Autodesk Inventor part; units mm, degrees
ref_plane "YZ Plane" through (0, 0, 0) normal (1, 0, 0) x (0, 1, 0)
ref_plane "XZ Plane" through (0, 0, 0) normal (0, 1, 0) x (-1, 0, 0)
ref_plane "XY Plane" through (0, 0, 0) normal (0, 0, 1) x (1, 0, 0)
sketch "Sketch1" plane through (0, 0, 0) normal (0, 0, 1) x (1, 0, 0)
  circle A0 centre (0, 0) radius 4.445
  dimension "d0" = 8.89
extrude "Extrusion1" add sketch "Sketch1" along normal blind 1.27
sketch "Sketch2" plane through (0, 0, 0) normal (0, 0, -1) x (-1, 0, 0)
  circle A0 centre (0, 0) radius 4.445
  circle A1 centre (0, 0) radius 1.27
  dimension "d3" = 2.54
extrude "Extrusion2" add sketch "Sketch2" along normal blind 1.27 contours A1
sketch "Sketch3" plane through (0, 0, 1.27) normal (0, 0, 1) x (1, 0, 0)
  circle A0 centre (0, 0) radius 4.445
  circle A1 centre (0, 0) radius 3.175
  dimension "d6" = 6.35
extrude "Extrusion3" add sketch "Sketch3" along normal blind 1.27 contours A1
sketch "Sketch4" plane through (0, 0, 2.54) normal (0, 0, 1) x (1, 0, 0)
  circle A0 centre (0, 0) radius 3.175
  line L0 (6.35, -9.525) -> (6.35, 9.525)
  line L1 (4.9582, 9.1002) -> (-14.9068, 3.0367)
  line L2 (-14.9068, -3.0367) -> (4.9582, -9.1002)
  arc A1 (7.808, -8.5899) -> (7.808, 8.5899) centre (1.27, 0) ccw
  arc A2 (-14.9068, 3.0367) -> (-14.9068, -3.0367) centre (-13.9799, 0) ccw
  arc A3 (7.808, 8.5899) -> (4.9582, 9.1002) centre (5.8851, 6.0635) ccw
  arc A4 (4.9582, -9.1002) -> (7.808, -8.5899) centre (5.8851, -6.0635) ccw
  point P0 (-24.8555, 0)
  dimension "d9" = 19.05
  dimension "d13" = 9.525
  dimension "d14" = 6.35
  dimension "d15" = 10.795
  dimension "d16" = 3.175
  dimension "d20" = 0
  dimension "d21" = 22.225
  dimension "d22" = 3.175
extrude "Extrusion4" add sketch "Sketch4" along normal blind 3.81 contours A0 | A4 L2 A2 L1 A3 L0 | L0 A3 A1 A4
properties part number "Knob 1764"
Check sheet for the modelled part. Datum: model origin and axes. Units: mm. A direction names the side the tool comes from. Round coordinates to 2 decimals unless told otherwise and drop trailing zeros. Write each loop counter-clockwise with the first axis right and the second up, starting at its lowest first coordinate (ties: lowest second). Pieces come first, ordered by that corner, then holes. Notation, with made-up numbers: (18, -8) - (29, -8) arc R31 ccw to (29, 24) - close; hole circle Ø10 at (58.5, 32.5). An arc over 180 degrees is marked (long way). Return JSON: item names as keys, results as strings.
Q1. Cross-section at B-B (y = 0). Record the boundary of the cut face in (x, z) (3 decimals).
Returned:
{"outline": "(-17.155, 2.54) - (-3.175, 2.54) - (-3.175, 1.27) - (-4.445, 1.27) - (-4.445, 0) - (-1.27, 0) - (-1.27, -1.27) - (1.27, -1.27) - (1.27, 0) - (4.445, 0) - (4.445, 1.27) - (3.175, 1.27) - (3.175, 2.54) - (12.065, 2.54) - (12.065, 6.35) - (-17.155, 6.35) - close"}
Q2. Depth check by flat-ended pin: P1, Ø1.5, axis at x = -5.5, y = -4, coming from the -Z side; P2, Ø4, axis at x = -5.5, y = 6.5, coming from the +Z side; P3, Ø8, axis at x = 0, y = 7, coming from the -Z side; P4, Ø1, axis at x = -12.5, z = 0.5, coming from the +Y side. Enter the tip coordinate at first touch or a pass-through.
Returned:
{"P1": "stops at z = 2.54", "P2": "stops at z = 6.35", "P3": "stops at z = 0", "P4": "passes through"}
Q3. Access from +Z, -Z, +X, -X, +Y, -Y to the whole of each face (thin tool, end or side, straight path). Record for faces 1 (the flat face through (-1.1, -0.9, 0)), 2 (the cylindrical face through (12.064, 0.139, 4.418)).
Returned:
{"face 1": "-Z", "face 2": "+Z, -Z, +X"}
Q4. Scan lines: L1, parallel to Z at x = -1.25, y = -1.5; L2, parallel to Z at x = 6.5, y = 5.25; L3, parallel to Z at x = 4.25, y = -0.25. Record each from-to range of solid material in increasing order. Write a range as from..to.
Returned:
{"L1": "z = 0..6.35", "L2": "z = 2.54..6.35", "L3": "z = 0..1.27, 2.54..6.35"}
Q5. Cross-section at A-A (x = -4). Record the boundary of the cut face in (y, z).
Returned:
{"outline": "(-6.37, 2.54) - (6.37, 2.54) - (6.37, 6.35) - (-6.37, 6.35) - close; (-1.94, 0) - (1.94, 0) - (1.94, 1.27) - (-1.94, 1.27) - close"}
Q6. Cross-section at D-D (z = 3.5). Record the boundary of the cut face in (x, y) (3 decimals), then the cut area to 3 significant figures.
Returned:
{"outline": "(-14.907, -3.037) - (4.958, -9.1) arc R3.175 ccw to (7.808, -8.59) arc R10.795 ccw to (7.808, 8.59) arc R3.175 ccw to (4.958, 9.1) - (-14.907, 3.037) arc R3.175 ccw to start", "area": "354 mm²"}
Q7. Draft check along Z on faces 3 (the flat face through (0, 0, 6.35)), 4 (the flat face through (2, -3, 1.27)), 5 (the cylindrical face through (-0.69, 3.1, 1.9)), 6 (the flat face through (-4.84, 6.11, 4.42)). Enter one of: released by +Z, released by -Z, zero draft, split by the parting line, or undercut.
Returned:
{"face 3": "released by +Z", "face 4": "undercut", "face 5": "undercut", "face 6": "zero draft"}
Q8. Cross-section at C-C (y = 4). Record the boundary of the cut face in (x, z).
Returned:
{"outline": "(-11.75, 2.54) - (11.3, 2.54) - (11.3, 6.35) - (-11.75, 6.35) - close; (-1.94, 0) - (1.94, 0) - (1.94, 1.27) - (-1.94, 1.27) - close"}
